Could you check a few things on this model? Use its own coordinates, in mm. A direction names the side the tool comes from. Give positions to 0.01 mm unless a question says otherwise; leave off trailing zeros. Loops run counter-clockwise (first coordinate to the right, second up) from the corner with the lowest first, then second, coordinate; pieces in that order, holes last. Notation, with made-up numbers: M 48,77.25 L 53,77.25 A21 ccw 53,115.25 Z; hole C 38,4.25 d9. An arc over 180 degrees is marked long. Use CSV: the item, a comma, the result in double quotes.
```python
from build123d import *

# Parameters (mm, degrees)
SKETCH1_R           = 2
BOSS_EXTRUDE1_DEPTH = 5
BOSS_EXTRUDE2_DEPTH = 10
CHAMFER2_SIZE       = 10


with BuildPart() as part:
    # Sketch1 → Boss-Extrude1 (new body)
    with BuildSketch(Plane.XY):
        with BuildLine():
            ThreePointArc((58.593094964, -62.917012913), (58.124418815, -35.115379165), (45.172708428, -10.510426525))
            Line((45.172708428, -10.510426525), (34.120235365, 2.132661237))
            Line((34.120235365, 2.132661237), (65.536970349, 88.4494312))
            ThreePointArc((65.536970349, 88.4494312), (66.199502533, 94.806221081), (62.474937186, 100))
            Line((62.474937186, 100), (55, 100))
            Line((55, 100), (-55, 100))
            Line((-55, 100), (-62.474937186, 100))
            ThreePointArc((-62.474937186, 100), (-66.199502533, 94.806221081), (-65.536970349, 88.4494312))
            Line((-65.536970349, 88.4494312), (-34.120235365, 2.132661237))
            Line((-34.120235365, 2.132661237), (-45.172708428, -10.510426525))
            ThreePointArc((-45.172708428, -10.510426525), (-58.124418815, -35.115379165), (-58.593094964, -62.917012913))
            Line((-58.593094964, -62.917012913), (-51.644303304, -94.437551937))
            ThreePointArc((-51.644303304, -94.437551937), (-50.278037542, -97.589552755), (-47.830276245, -100))
            Line((-47.830276245, -100), (-40.355339059, -100))
            Line((-40.355339059, -100), (40.355339059, -100))
            Line((40.355339059, -100), (47.830276245, -100))
            ThreePointArc((47.830276245, -100), (50.278037542, -97.589552755), (51.644303304, -94.437551937))
            Line((51.644303304, -94.437551937), (58.593094964, -62.917012913))
        make_face()
        with Locations((-42.855339059, -92.5)):
            Circle(SKETCH1_R, mode=Mode.SUBTRACT)
        with Locations((42.855339059, -92.5)):
            Circle(SKETCH1_R, mode=Mode.SUBTRACT)
        with Locations((-57.5, 92.5)):
            Circle(SKETCH1_R, mode=Mode.SUBTRACT)
        with Locations((57.5, 92.5)):
            Circle(SKETCH1_R, mode=Mode.SUBTRACT)
    extrude(amount=BOSS_EXTRUDE1_DEPTH)

    # Sketch2 → Boss-Extrude2 (add)
    with BuildSketch(Plane(origin=(0, 0, 0), x_dir=(-1, 0, 0), z_dir=(0, 0, -1))):
        with BuildLine():
            Line((-25.870507592, 10.166666667), (-24.253462846, 5.723872742))
            ThreePointArc((-24.253462846, 5.723872742), (-23.669056818, 3.144030102), (-23.747944524, 0.5))
            Line((-23.747944524, 0.5), (23.747944524, 0.5))
            ThreePointArc((23.747944524, 0.5), (23.669056818, 3.144030102), (24.253462846, 5.723872742))
            Line((24.253462846, 5.723872742), (25.870507592, 10.166666667))
            Line((25.870507592, 10.166666667), (-25.870507592, 10.166666667))
        make_face()
    extrude(amount=BOSS_EXTRUDE2_DEPTH)

    # Chamfer2
    # the kernel refuses this chamfer: 10 mm, written as the material it takes off along each edge
    with BuildSketch(Plane(origin=(-51.587337472, 10.166666667, -10), x_dir=(0, 0.027495876610586317, 0.9996219169112968), z_dir=(1, 0, 0))) as chamfer2_piece_1_section:
        Polygon((CHAMFER2_SIZE * 0.999621916911, CHAMFER2_SIZE * 0.0274958766106), (-CHAMFER2_SIZE * 0.0274958766106, CHAMFER2_SIZE * 0.999621916911), (0, 0), align=None)
    chamfer2_piece_1 = extrude(amount=103.174674944, mode=Mode.PRIVATE)
    chamfer2_piece_1 = split(chamfer2_piece_1, bisect_by=Plane(origin=(0, 6.862625123, 0), z_dir=(0, 0, -1)), keep=Keep.TOP, mode=Mode.PRIVATE)
    add(chamfer2_piece_1, mode=Mode.SUBTRACT)


solid = part.part
```
1. I'm going to push flat-ended pins straight in: pin 1 Ø3 at (y, z) = (4, -7.5) entering from +X; pin 2 Ø1.5 at (y, z) = (10, 2.5) entering from +X; pin 3 Ø5 at (x, z) = (-10, -5.5) entering from -Y; pin 4 Ø3 at (y, z) = (54, -3) entering from +X. Where does each tip first touch, or does it pass through?
Outcome:
pin 1,"x = 23.82"
pin 2,"x = 37.26"
pin 3,"y = 0.5"
pin 4,"through"
2. I want a section at A-A, the plane y = 92.5. List the corners of the cut face in (x, z) for me, then the cut area to 3 significant figures.
Outcome:
outline,"M -66.5,0 L -59.5,0 L -59.5,5 L -66.5,5 Z; M -55.5,0 L 55.5,0 L 55.5,5 L -55.5,5 Z; M 59.5,0 L 66.5,0 L 66.5,5 L 59.5,5 Z"
area,"625 mm2"
3. Which directions (+Z, -Z, +X, -X, +Y, -Y) give clear straight access to the entire face, cutting with the end or side of a thin tool? Please do faces 4 (the face through (24.714, 6.989, -1.203)), 5 (the face through (49.61, 44.69, 2.46)), 6 (the face through (-23.627, 2.519, -3.692)).
Outcome:
face 4,"-Z, +X, -Y"
face 5,"+Z, -Z, +X"
face 6,"-Z, -X"
4. I want a section at C-C, the plane y = -92.5. List the corners of the cut face in (x, z) for me.
Outcome:
outline,"M -52.07,0 L -44.86,0 L -44.86,5 L -52.07,5 Z; M -40.86,0 L 40.86,0 L 40.86,5 L -40.86,5 Z; M 44.86,0 L 52.07,0 L 52.07,5 L 44.86,5 Z"
5. I want a section at D-D, the plane z = -7. List the corners of the cut face in (x, y) for me, then the cut area to 3 significant figures.
Outcome:
outline,"M -23.75,0.5 L 23.75,0.5 A10.5 cw 23.67,3.17 L -23.67,3.17 A10.5 cw Z"
area,"126 mm2"
6. I want a section at B-B, the plane x = -2. List the corners of the cut face in (y, z) for me, then the cut area to 3 significant figures.
Outcome:
outline,"M -100,0 L 0.5,0 L 0.5,-9.67 L 10.17,0 L 100,0 L 100,5 L -100,5 Z"
area,"1,050 mm2"
7. If we mould it in two halves opening along X, with no side actions, what happens to faces 1 (the face through (-43.116, -90.517, 2.465)), 2 (the face through (23.63, 2.59, -3.69)), 3 (the face through (-39.57, -4.1, 2.46))? For each: +X half, -X half, draft (parallel to the pull), parting line (faces both ways), or undercut.
Outcome:
face 1,"undercut"
face 2,"+X half"
face 3,"-X half"
8. Please list where these lines run through material, in increasing order: line 1 (Z direction, x = -58.5, y = -40); line 2 (Y direction, x = 5, z = -0.5); line 3 (Y direction, x = -20, z = -2.25).
Outcome:
line 1,"0 to 5"
line 2,"0.5 to 9.67"
line 3,"0.5 to 7.92"
